Drawing for the job (mm, zero at the part's lowest x, y, z). Coordinates: 2 decimals unless noted, no trailing zeros. Order: outer loops, then holes, each group sorted by start corner. A loop starts at its lowest first (then second) coordinate and runs counter-clockwise, first axis right, second up. Notation, with made-up numbers: M -6,-32 L 0,-32 A18 cw 0,-28 Z; hole C 75.25,-13.75 d5. An arc over 180 degrees is marked long. Write item = value, one per line. Start each with the question number.
Q1. Band-saw the part on D-D on y = 10.75. Write the cut outline in (x, z).
Q2. Band-saw the part on A-A on y = 6.35. Write the cut outline in (x, z).
Q3. Pull direction Y, two halves, no side cores. Call the marked faces 1, 2 and 3: released by +Y, released by -Y, zero draft, split by the parting line, or undercut.
Q4. Pin check, flat tip, straight feed: P1, Ø2.5, axis at x = 5.5, z = 6.35, coming from the -Y side (3 decimals). Stop position of the tip, or through.
Q5. Band-saw the part on B-B on x = 59.5. Write the cut outline in (y, z), plus the area to 3 significant figures.
Q6. Drill centre lines: probe 1 along X at (y, z) = (6.5, 10.5); probe 2 along X at (y, z) = (3, 6.35); probe 3 along Z at (x, y) = (5.5, 2.75). Where is each one in solid material? Low to high.
Q7. Band-saw the part on C-C on z = 6.35. Write the cut outline in (x, y), plus the area to 3 significant figures.
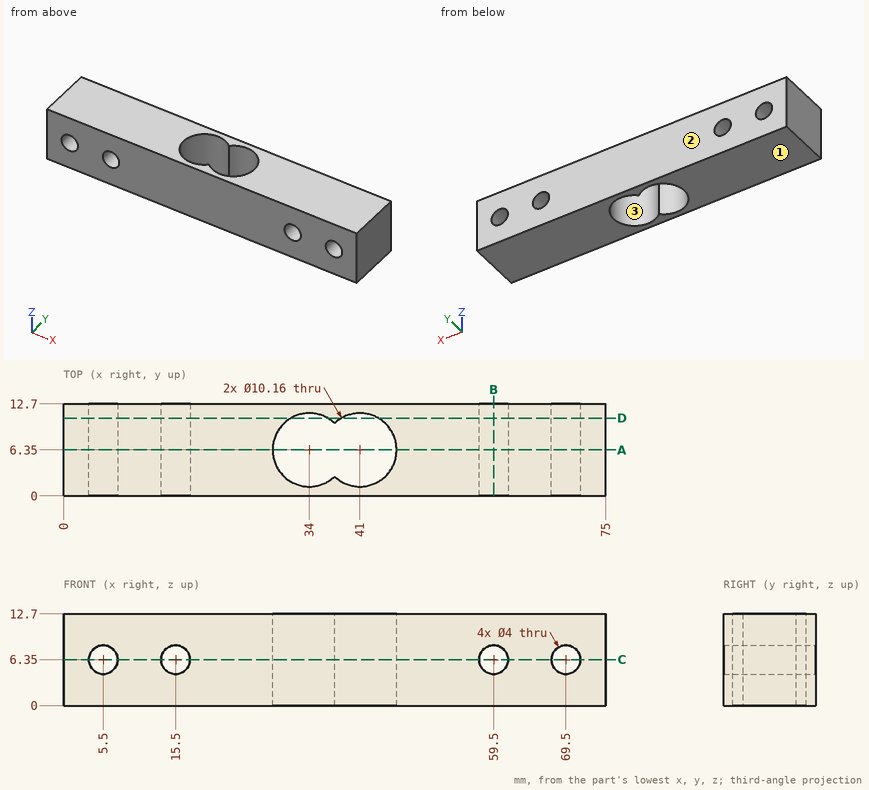
Recorded:
q1.outline = M 0,0 L 31.46,0 L 31.46,12.7 L 0,12.7 Z; M 36.54,0 L 38.46,0 L 38.46,12.7 L 36.54,12.7 Z; M 43.54,0 L 75,0 L 75,12.7 L 43.54,12.7 Z; hole C 5.5,6.35 d4; hole C 15.5,6.35 d4; hole C 59.5,6.35 d4; hole C 69.5,6.35 d4
q2.outline = M 0,0 L 28.92,0 L 28.92,12.7 L 0,12.7 Z; M 46.08,0 L 75,0 L 75,12.7 L 46.08,12.7 Z; hole C 5.5,6.35 d4; hole C 15.5,6.35 d4; hole C 59.5,6.35 d4; hole C 69.5,6.35 d4
q3.face_1 = zero draft
q3.face_2 = released by +Y
q3.face_3 = undercut
q4.P1 = through
q5.outline = M 0,0 L 12.7,0 L 12.7,4.35 L 0,4.35 Z; M 0,8.35 L 12.7,8.35 L 12.7,12.7 L 0,12.7 Z
q5.area = 110 mm2
q6.probe_1 = 0 to 28.92, 46.08 to 75
q6.probe_2 = 0 to 3.5, 7.5 to 13.5, 17.5 to 30.18, 44.82 to 57.5, 61.5 to 67.5, 71.5 to 75
q6.probe_3 = 0 to 4.35, 8.35 to 12.7
q7.outline = M 0,0 L 3.5,0 L 3.5,12.7 L 0,12.7 Z; M 7.5,0 L 13.5,0 L 13.5,12.7 L 7.5,12.7 Z; M 17.5,0 L 57.5,0 L 57.5,12.7 L 17.5,12.7 Z; M 61.5,0 L 67.5,0 L 67.5,12.7 L 61.5,12.7 Z; M 71.5,0 L 75,0 L 75,12.7 L 71.5,12.7 Z; hole M 37.5,2.67 A5.08 ccw long 37.5,10.03 A5.08 ccw long Z
q7.area = 603 mm2
